```python
from build123d import *

# Parameters (mm, degrees)
ESQUISSE1_R                  = 2.5
BOSS_EXTRU_1_DEPTH           = 5
ESQUISSE2_R                  = 1.25
ENL_V_MAT_EXTRU_1_DEPTH      = 11
R_P_TITION_CIRCULAIRE1_COUNT = 3
ESQUISSE4_R                  = 2
ENL_V_MAT_EXTRU_3_DEPTH      = 11
ESQUISSE5_W                  = 60.3
ESQUISSE5_H                  = 80.3
ESQUISSE5_W_2                = 39.7
ESQUISSE5_H_2                = 59.7
ENL_V_MAT_EXTRU_4_DEPTH      = 8
ESQUISSE6_R                  = 6.325
ESQUISSE6_R_2                = 3.325
BOSS_EXTRU_2_DEPTH           = 10
ENL_V_MAT_EXTRU_5_DEPTH      = 31.04
R_P_TITION_CIRCULAIRE2_COUNT = 3


with BuildPart() as part:
    # Esquisse1 → Boss.-Extru.1 (new body, symmetric)
    with BuildSketch(Plane(origin=(0, 0, 0), x_dir=(1, 0, 0), z_dir=(0, 1, 0))):
        Polygon((-10, 79.372539332), (10, 79.372539332), (73.738635424, -31.026015628), (63.738635424, -48.346523704), (-63.738635424, -48.346523704), (-73.738635424, -31.026015628), align=None)
        Circle(ESQUISSE1_R, mode=Mode.SUBTRACT)
    extrude(amount=BOSS_EXTRU_1_DEPTH, both=True)

    # Esquisse2 → Enlèv. mat.-Extru.1 (cut, through all)
    with BuildSketch(Plane(origin=(0, 5, 0), x_dir=(1, 0, 0), z_dir=(0, 1, 0))):
        with Locations((-62.685117852, -36.191269666)):
            Circle(ESQUISSE2_R)
        with Locations((-47.910724463, -27.661269666)):
            Circle(ESQUISSE2_R)
    enl_v_mat_extru_1 = extrude(amount=-ENL_V_MAT_EXTRU_1_DEPTH, mode=Mode.SUBTRACT)

    # Répétition circulaire1: Enlèv. mat.-Extru.1 ×3 about axis
    r_p_tition_circulaire1_axis = Axis((0, 0, 0), (0, 1, 0))
    for i in range(1, R_P_TITION_CIRCULAIRE1_COUNT):
        add(enl_v_mat_extru_1.rotate(r_p_tition_circulaire1_axis, i * 360 / R_P_TITION_CIRCULAIRE1_COUNT), mode=Mode.SUBTRACT)

    # Esquisse4 → Enlèv. mat.-Extru.3 (cut, through all)
    with BuildSketch(Plane.XZ.offset(5)):
        with Locations((0, -30.32)):
            Circle(ESQUISSE4_R)
        with Locations((0, 39.68)):
            Circle(ESQUISSE4_R)
        with Locations((25, 4.68)):
            Circle(ESQUISSE4_R)
        with Locations((-25, 4.68)):
            Circle(ESQUISSE4_R)
    extrude(amount=-ENL_V_MAT_EXTRU_3_DEPTH, mode=Mode.SUBTRACT)

    # Esquisse5 → Enlèv. mat.-Extru.4 (cut)
    with BuildSketch(Plane.XZ.offset(5)):
        with Locations((0, 4.68)):
            Rectangle(ESQUISSE5_W, ESQUISSE5_H)
        with Locations((0, 4.68)):
            Rectangle(ESQUISSE5_W_2, ESQUISSE5_H_2, mode=Mode.SUBTRACT)
    extrude(amount=-ENL_V_MAT_EXTRU_4_DEPTH, mode=Mode.SUBTRACT)

    # Esquisse6 → Boss.-Extru.2 (add)
    with BuildSketch(Plane.XZ.offset(5)):
        with Locations((0, 20.18)):
            Circle(ESQUISSE6_R)
        with Locations((0, 20.18)):
            Circle(ESQUISSE6_R_2, mode=Mode.SUBTRACT)
    extrude(amount=BOSS_EXTRU_2_DEPTH)

    # Esquisse7 → Enlèv. mat.-Extru.5 (cut)
    with BuildSketch(Plane(origin=(-68.738635424, 0, 39.686269666), x_dir=(0.5, 0, 0.866025404), z_dir=(-0.866025404, 0, 0.5))):
        Polygon((-2.65, 5), (-6.38, -3), (6.38, -3), (2.65, 5), align=None)
    enl_v_mat_extru_5 = extrude(amount=-ENL_V_MAT_EXTRU_5_DEPTH, mode=Mode.SUBTRACT)

    # Répétition circulaire2: Enlèv. mat.-Extru.5 ×3 about axis
    r_p_tition_circulaire2_axis = Axis((0, 0, 0), (0, 1, 0))
    for i in range(1, R_P_TITION_CIRCULAIRE2_COUNT):
        add(enl_v_mat_extru_5.rotate(r_p_tition_circulaire2_axis, i * 360 / R_P_TITION_CIRCULAIRE2_COUNT), mode=Mode.SUBTRACT)


solid = part.part
```
Build history of the part. All positions in model axes, mm. A direction names the side the tool comes from. Give positions to 0.01 mm unless a question says otherwise; leave off trailing zeros. Loops run counter-clockwise (first coordinate to the right, second up) from the corner with the lowest first, then second, coordinate; pieces in that order, holes last. Notation, with made-up numbers: (19.25, 22.25) -> (27.25, 22.25) arc R18 cw to (27.25, 56.25) -> close; hole circle Ø3 at (38.5, -33). An arc over 180 degrees is marked (long way). One line per question, with ' | ' between items. Start each with the question number.
1) Cut at D-D (y = -9.25). Give the cut face in (x, z) (3 decimals), plus the area to 3 significant figures.
2) Pin check, flat tips, straight feed: pin 1 (9 mm diameter, centred on y = -2, z = 22, fed in from -X); pin 2 (12 mm diameter, centred on y = 3, z = -7.5, fed in from -X); pin 3 (1.5 mm diameter, centred on y = -1, z = -59, fed in from +X). Stop position of each tip, or through.
3) 3-axis set-ups, long thin cutter, end or side, ignore diameter. For faces 5 (the flat face through (-19.85, -1, 4)), 6 (the flat face through (41.42, 0.07, -24.95)), 7 (the flat face through (0, 0, -48.333)), 8 (the flat face through (41.813, 0.167, 24.244)): which of +Z, -Z, +X, -X, +Y, -Y reach the whole face in a straight line?
4) Cut at B-B (z = 0). Give the cut face in (x, y).
5) Cut at A-A (x = 25). Give the cut face in (y, z), plus the area to 3 significant figures.
6) Probe L1, parallel to Z at x = 9.5, y = -4.25; L2, parallel to X at y = -3.25, z = 32; L3, parallel to Z at x = -5, y = -2.25. List the from-to ranges inside material, lowest first.
7) Two-plate mould, pull along Y, no slides. Class faces 1 (the flat face through (0, -5, 20)), 2 (the cylindrical face through (-0.82, -9.93, 26.45)), 3 (the flat face through (1, 5, 12)), 4 (the flat face through (4.489, 1.056, -64.07)): released by +Y, released by -Y, zero draft, split by the parting line, or undercut.
8) Cut at C-C (y = -1). Give the cut face in (x, z).
Return value:
1) outline: circle Ø12.65 at (0, 20.18); hole circle Ø6.65 at (0, 20.18) | area: 90.9 mm^2
2) pin 1: x = -71.13 | pin 2: x = -54.96 | pin 3: x = 22.2
3) face 5: -Y | face 6: -Z, +X, +Y, -Y | face 7: -Z | face 8: none
4) outline: (-55.83, -5) -> (-30.15, -5) -> (-30.15, 3) -> (-19.85, 3) -> (-19.85, -5) -> (-2.5, -5) -> (-2.5, 5) -> (-55.83, 5) -> close; (2.5, -5) -> (19.85, -5) -> (19.85, 3) -> (30.15, 3) -> (30.15, -5) -> (55.83, -5) -> (55.83, 5) -> (2.5, 5) -> close
5) outline: (-5, -53.39) -> (5, -53.39) -> (5, 2.68) -> (3, 2.68) -> (3, -35.47) -> (-5, -35.47) -> close; (-5, 44.83) -> (3, 44.83) -> (3, 6.68) -> (5, 6.68) -> (5, 48.35) -> (-5, 48.35) -> close | area: 367 mm^2
6) L1: -79.37 to -35.47, -25.17 to 34.53, 44.83 to 48.35 | L2: -73.18 to -30.15, -19.85 to 19.85, 30.15 to 73.18 | L3: -48.33 to -35.47, -25.17 to 34.53, 44.83 to 48.35
7) face 1: released by -Y | face 2: zero draft | face 3: released by +Y | face 4: undercut
8) outline: (-73.74, 31.03) -> (-10, -79.37) -> (-5.45, -79.37) -> (-5.45, -48.33) -> (5.45, -48.33) -> (5.45, -79.37) -> (10, -79.37) -> (73.74, 31.03) -> (71.46, 34.97) -> (44.58, 19.45) -> (39.13, 28.88) -> (66.01, 44.4) -> (63.74, 48.35) -> (-63.74, 48.35) -> (-66.01, 44.4) -> (-39.13, 28.88) -> (-44.58, 19.45) -> (-71.46, 34.97) -> close; (-19.85, -25.17) -> (19.85, -25.17) -> (19.85, 34.53) -> (-19.85, 34.53) -> close; hole (-30.15, -35.47) -> (30.15, -35.47) -> (30.15, 44.83) -> (-30.15, 44.83) -> close; hole circle Ø5 at (0, 0)
